Part model, mm, in its own coordinate system. A direction names the side the tool comes from. Round coordinates to 2 decimals unless told otherwise and drop trailing zeros. Loops run counter-clockwise (first coordinate to the right, second up) from the corner with the lowest first, then second, coordinate; pieces in that order, holes last. Notation, with made-up numbers: (52.25, 36.25) -> (57.25, 36.25) arc R15 cw to (57.25, 51.25) -> close; hole circle Ø6 at (59, -23). An arc over 180 degrees is marked (long way). Answer as a JSON object with one key per item and string values. Group by question number.
from build123d import *

# Parameters (mm, degrees)
SKETCH1_W                = 140
SKETCH1_H                = 70
BOSS_EXTRUDE1_DEPTH      = 30
SKETCH2_W                = 130
SKETCH2_H                = 60
CUT_EXTRUDE1_DEPTH       = 25
SKETCH3_W                = 5
SKETCH3_H                = 5.715
CUT_EXTRUDE2_DEPTH       = 25
SKETCH4_W                = 20
SKETCH4_H                = 10
CUT_EXTRUDE6_DEPTH       = 25
M3_CLEARANCE_HOLE1_D     = 3.6
M3_CLEARANCE_HOLE1_DEPTH = 5
M3_CLEARANCE_HOLE1_TIP   = 1.081549114


with BuildPart() as part:
    # Sketch1 → Boss-Extrude1 (new body)
    with BuildSketch(Plane(origin=(0, 0, 0), x_dir=(1, 0, 0), z_dir=(0, 1, 0))):
        with Locations((70, 35)):
            Rectangle(SKETCH1_W, SKETCH1_H)
    extrude(amount=BOSS_EXTRUDE1_DEPTH)

    # Sketch2 → Cut-Extrude1 (cut)
    with BuildSketch(Plane(origin=(0, 30, 0), x_dir=(1, 0, 0), z_dir=(0, 1, 0))):
        with Locations((70, 35)):
            Rectangle(SKETCH2_W, SKETCH2_H)
    extrude(amount=-CUT_EXTRUDE1_DEPTH, mode=Mode.SUBTRACT)

    # Sketch3 → Cut-Extrude2 (cut)
    with BuildSketch(Plane.XZ):
        with BuildLine():
            ThreePointArc((22.5, -15), (21.767766953, -13.232233047), (20, -12.5))
            Line((20, -12.5), (20, -15))
            Line((20, -15), (20, -17.5))
            ThreePointArc((20, -17.5), (21.767766953, -16.767766953), (22.5, -15))
        make_face()
        with BuildLine():
            ThreePointArc((45.533822472, -15), (32.389100257, -9.555277785), (37.833822472, -22.7))
            ThreePointArc((37.833822472, -22.7), (43.278544687, -20.444722215), (45.533822472, -15))
        make_face()
        Polygon((57.017644944, -20), (62.017644944, -20), (69.717644944, -20), (69.717644944, -8.57), (57.017644944, -8.57), (57.017644944, -15), align=None)
        Polygon((69.717644944, -50), (62.017644944, -50), (57.017644944, -50), (57.017644944, -61.43), (69.717644944, -61.43), align=None)
        with Locations((59.517644944, -32.1425)):
            Rectangle(SKETCH3_W, SKETCH3_H)
        with Locations((59.517644944, -37.8575)):
            Rectangle(SKETCH3_W, SKETCH3_H)
        with BuildLine():
            ThreePointArc((45.533822472, -55), (43.278544687, -49.555277785), (37.833822472, -47.3))
            ThreePointArc((37.833822472, -47.3), (32.389100257, -60.444722215), (45.533822472, -55))
        make_face()
        with BuildLine():
            ThreePointArc((37.833822472, -27.3), (32.389100257, -29.555277785), (30.133822472, -35))
            Line((30.133822472, -35), (37.833822472, -35))
            Line((37.833822472, -35), (37.833822472, -27.3))
        make_face()
        with BuildLine():
            Line((37.833822472, -35), (30.133822472, -35))
            ThreePointArc((30.133822472, -35), (32.389100257, -40.444722215), (37.833822472, -42.7))
            Line((37.833822472, -42.7), (37.833822472, -35))
        make_face()
        with BuildLine():
            ThreePointArc((22.5, -55), (21.767766953, -53.232233047), (20, -52.5))
            Line((20, -52.5), (20, -57.5))
            ThreePointArc((20, -57.5), (21.767766953, -56.767766953), (22.5, -55))
        make_face()
        with BuildLine():
            Line((20, -57.5), (20, -52.5))
            ThreePointArc((20, -52.5), (17.5, -55), (20, -57.5))
        make_face()
        with BuildLine():
            ThreePointArc((22.5, -35), (21.767766953, -33.232233047), (20, -32.5))
            Line((20, -32.5), (20, -35))
            Line((20, -35), (22.5, -35))
        make_face()
        with BuildLine():
            Line((20, -35), (20, -32.5))
            ThreePointArc((20, -32.5), (17.5, -35), (20, -37.5))
            Line((20, -37.5), (20, -35))
        make_face()
        with BuildLine():
            Line((20, -15), (20, -12.5))
            ThreePointArc((20, -12.5), (17.5, -15), (20, -17.5))
            Line((20, -17.5), (20, -15))
        make_face()
        with BuildLine():
            Line((22.5, -35), (20, -35))
            Line((20, -35), (20, -37.5))
            ThreePointArc((20, -37.5), (21.767766953, -36.767766953), (22.5, -35))
        make_face()
        with BuildLine():
            Line((37.833822472, -27.3), (37.833822472, -35))
            Line((37.833822472, -35), (45.533822472, -35))
            ThreePointArc((45.533822472, -35), (43.278544687, -29.555277785), (37.833822472, -27.3))
        make_face()
        with BuildLine():
            Line((45.533822472, -35), (37.833822472, -35))
            Line((37.833822472, -35), (37.833822472, -42.7))
            ThreePointArc((37.833822472, -42.7), (43.278544687, -40.444722215), (45.533822472, -35))
        make_face()
        Polygon((62.017644944, -29.285), (62.017644944, -35), (62.017644944, -40.715), (68.367644944, -40.715), (69.717644944, -40.715), (69.717644944, -29.285), (68.367644944, -29.285), align=None)
    extrude(amount=-CUT_EXTRUDE2_DEPTH, mode=Mode.SUBTRACT)

    # Sketch4 → Cut-Extrude6 (cut)
    with BuildSketch(Plane(origin=(140, 0, 0), x_dir=(0, 0, -1), z_dir=(1, 0, 0))):
        with Locations((15, 10)):
            Rectangle(SKETCH4_W, SKETCH4_H)
    extrude(amount=-CUT_EXTRUDE6_DEPTH, mode=Mode.SUBTRACT)

    # M3 Clearance Hole1
    with Locations(Plane(origin=(0, 30, 0), x_dir=(1, 0, 0), z_dir=(0, 1, 0))):
        with Locations((2.5, 2.5), (2.5, 67.5), (137.5, 67.5), (137.5, 2.5)):
            Hole(M3_CLEARANCE_HOLE1_D / 2, depth=M3_CLEARANCE_HOLE1_DEPTH)
            with Locations((0, 0, -(M3_CLEARANCE_HOLE1_DEPTH + M3_CLEARANCE_HOLE1_TIP / 2))):  # 118° drill point
                Cone(0, M3_CLEARANCE_HOLE1_D / 2, M3_CLEARANCE_HOLE1_TIP, mode=Mode.SUBTRACT)


solid = part.part
Item 1: Band-saw the part on C-C, the plane y = 3. Count the separate pieces of the cut face and the enclosed holes in it, plus the area to 3 significant figures.
Item 2: Two-plate mould, pull along Z, no slides. Class faces 1 (the face through (138, 15, -15)), 2 (the face through (0, 15, -35)): pulls with the +Z half, pulls with the -Z half, needs draft (parallel to the pull), parting line crosses it, or undercut.
Item 3: Band-saw the part on B-B, the plane x = 66. List the corners of the cut face in (y, z) (3 decimals), plus the area to 3 significant figures.
Item 4: Band-saw the part on A-A, the plane y = 20.75. List the corners of the cut face in (x, z), plus the area to 3 significant figures.
Item 5: Drill centre lines: line 1 (X direction, y = 28.2, z = -67.5); line 2 (X direction, y = 1.05, z = -15); line 3 (Z direction, x = 2.5, y = 27.4). Where is each one in solid material? Low to high.
Item 6: Which spindle directions (+Z, -Z, +X, -X, +Y, -Y) get a long thin tool onto all of the face, cutting with end or side? Do faces 3 (the face through (135, 18, -41)), 4 (the face through (70, 30, -66)), 5 (the face through (63, 2, -20)). Say none if no direction does.
Item 7: Drop a flat-ended pin along its axis: pin 1 Ø10 at (x, z) = (74.5, -50) entering from +Y. Give the stop position or say it passes through.
Item 8: Band-saw the part on D-D, the plane z = -11. List the corners of the cut face in (x, y).
Entries:
{
 "1": {"separate pieces": "1", "enclosed holes": "9", "area": "8,750 mm²"},
 "2": {"face 1": "undercut", "face 2": "needs draft"},
 "3": {"outline": "(0, -70) -> (30, -70) -> (30, -65) -> (5, -65) -> (5, -61.43) -> (0, -61.43) -> close; (0, -50) -> (5, -50) -> (5, -40.715) -> (0, -40.715) -> close; (0, -29.285) -> (5, -29.285) -> (5, -20) -> (0, -20) -> close; (0, -8.57) -> (5, -8.57) -> (5, -5) -> (30, -5) -> (30, 0) -> (0, 0) -> close", "area": "429 mm²"},
 "4": {"outline": "(0, -70) -> (140, -70) -> (140, 0) -> (0, 0) -> close; hole (5, -65) -> (135, -65) -> (135, -5) -> (5, -5) -> close", "area": "2,000 mm²"},
 "5": {"line 1": "0 to 0.7, 4.3 to 135.7, 139.3 to 140", "line 2": "0 to 17.5, 22.5 to 30.13, 45.53 to 57.02, 69.72 to 140", "line 3": "-70 to -69.3, -65.7 to -4.3, -0.7 to 0"},
 "6": {"face 3": "+Y", "face 4": "+Z, -Z, +X, -X, +Y", "face 5": "+Y, -Y"},
 "7": {"pin 1": "y = 5"},
 "8": {"outline": "(0, 0) -> (31.25, 0) -> (31.25, 5) -> (5, 5) -> (5, 30) -> (0, 30) -> close; (44.41, 0) -> (57.02, 0) -> (57.02, 5) -> (44.41, 5) -> close; (69.72, 0) -> (140, 0) -> (140, 5) -> (69.72, 5) -> close; (135, 15) -> (140, 15) -> (140, 30) -> (135, 30) -> close"}
}
